from build123d import *

# Parameters (mm, degrees)
BOSS_EXTRUDE1_DEPTH = 7.77


with BuildPart() as part:
    # Sketch1 → Boss-Extrude1 (new body)
    # profile 1 of 5: a face of its own
    with BuildSketch(Plane.XY):
        with BuildLine():
            ThreePointArc((3.404182759, -40.079440399), (3.403839221, -40.127801725), (3.402808675, -40.176153289))
            ThreePointArc((3.402808675, -40.176153289), (5.967670482, -39.875923927), (8.508052822, -39.412122972))
            ThreePointArc((8.508052822, -39.412122972), (35.574552979, -18.977712726), (37.472579791, 14.883150333))
            ThreePointArc((37.472579791, 14.883150333), (36.442962914, 17.251459476), (35.263848757, 19.548999228))
            ThreePointArc((35.263848757, 19.548999228), (30.43912953, 20.428209113), (31.453728524, 25.226283157))
            ThreePointArc((31.453728524, 25.226283157), (29.774333348, 27.188075947), (27.972797119, 29.038337096))
            ThreePointArc((27.972797119, 29.038337096), (18.347193458, 35.903800526), (7.14399719, 39.682057711))
            ThreePointArc((7.14399719, 39.682057711), (4.589484945, 40.057945878), (2.016151733, 40.269560864))
            ThreePointArc((2.016151733, 40.269560864), (2.020874049, 40.165888855), (2.022448638, 40.062121295))
            ThreePointArc((2.022448638, 40.062121295), (-1.382077907, 36.642156299), (-4.817411346, 40.031174701))
            ThreePointArc((-4.817411346, 40.031174701), (-7.369742742, 39.640752918), (-9.891851642, 39.087768817))
            ThreePointArc((-9.891851642, 39.087768817), (-34.597565404, 20.705334291), (-39.122221714, -9.7546998))
            ThreePointArc((-39.122221714, -9.7546998), (-38.417536694, -12.239087971), (-37.555259765, -14.673270392))
            ThreePointArc((-37.555259765, -14.673270392), (-34.193471955, -14.769982316), (-32.539881663, -17.698567233))
            ThreePointArc((-32.539881663, -17.698567233), (-33.081813677, -19.546068243), (-34.535867272, -20.808081887))
            ThreePointArc((-34.535867272, -20.808081887), (-33.133010631, -22.976205225), (-31.594239644, -25.05007827))
            ThreePointArc((-31.594239644, -25.05007827), (-21.298252211, -34.235754012), (-8.508052822, -39.412122972))
            ThreePointArc((-8.508052822, -39.412122972), (-5.967670482, -39.875923927), (-3.402808675, -40.176153289))
            ThreePointArc((-3.402808675, -40.176153289), (-0.048361325, -36.675601178), (3.404182759, -40.079440399))
        make_face()
        with BuildLine():
            ThreePointArc((-22.494419384, -11.066975129), (-5.681299846, 24.417200372), (25.069440399, 0))
            ThreePointArc((25.069440399, 0), (5.681299846, -24.417200372), (-22.494419384, -11.066975129))
        make_face(mode=Mode.SUBTRACT)
    # profile 2 of 5: a face of its own
    with BuildSketch(Plane.XY):
        with BuildLine():
            ThreePointArc((35.263848757, 19.548999228), (36.442962914, 17.251459476), (37.472579791, 14.883150333))
            ThreePointArc((37.472579791, 14.883150333), (40.378310636, 27.098559849), (27.972797119, 29.038337096))
            ThreePointArc((27.972797119, 29.038337096), (29.774333348, 27.188075947), (31.453728524, 25.226283157))
            ThreePointArc((31.453728524, 25.226283157), (34.9303084, 25.328891825), (36.69889556, 22.334023609))
            ThreePointArc((36.69889556, 22.334023609), (36.319038644, 20.767521125), (35.263848757, 19.548999228))
        make_face()
    # profile 3 of 5: a face of its own
    with BuildSketch(Plane.XY):
        with BuildLine():
            ThreePointArc((2.016151733, 40.269560864), (4.589484945, 40.057945878), (7.14399719, 39.682057711))
            ThreePointArc((7.14399719, 39.682057711), (-1.695633435, 48.606923637), (-9.891851642, 39.087768817))
            ThreePointArc((-9.891851642, 39.087768817), (-7.369742742, 39.640752918), (-4.817411346, 40.031174701))
            ThreePointArc((-4.817411346, 40.031174701), (-1.516784191, 43.480042232), (2.016151733, 40.269560864))
        make_face()
    # profile 4 of 5: a face of its own
    with BuildSketch(Plane.XY):
        with BuildLine():
            ThreePointArc((-39.122221714, -9.7546998), (-43.631335255, -21.474193014), (-31.594239644, -25.05007827))
            ThreePointArc((-31.594239644, -25.05007827), (-33.133010631, -22.976205225), (-34.535867272, -20.808081887))
            ThreePointArc((-34.535867272, -20.808081887), (-39.028605211, -19.208850623), (-37.555259765, -14.673270392))
            ThreePointArc((-37.555259765, -14.673270392), (-38.417536694, -12.239087971), (-39.122221714, -9.7546998))
        make_face()
    # profile 5 of 5: a face of its own
    with BuildSketch(Plane.XY):
        with BuildLine():
            ThreePointArc((8.508052822, -39.412122972), (5.967670482, -39.875923927), (3.402808675, -40.176153289))
            ThreePointArc((3.402808675, -40.176153289), (0, -43.483623159), (-3.402808675, -40.176153289))
            ThreePointArc((-3.402808675, -40.176153289), (-5.967670482, -39.875923927), (-8.508052822, -39.412122972))
            ThreePointArc((-8.508052822, -39.412122972), (0, -48.613623159), (8.508052822, -39.412122972))
        make_face()
    extrude(amount=BOSS_EXTRUDE1_DEPTH)

    # Fillet1
    # a fillet whose section is not a circle: 5 mm, written as the material it adds along each edge (its section moved 0.00015 mm through the faces so that the kernel can cut it)
    with BuildSketch(Plane(origin=(27.972797119, 29.038337096, 0), x_dir=(-0.7478052572443031, 0.6639181404644565, 0), z_dir=(0, 0, 1))) as fillet1_piece_1:
        with BuildLine():
            Bezier((3.27455803, 0), (0.443727696, -0.114917188), (-0.912581333, -2.602331942), weights=[1, 0.435020662, 1])
            Line((-0.912581333, -2.602331942), (-1.000377754, -2.554459315))
            ThreePointArc((-1.000377754, -2.554459315), (-0.444974343, -1.30513366), (-0.098468347, 0.017435156))
            Line((-0.098468347, 0.017435156), (0.004065293, 0.099917333))
            ThreePointArc((0.004065293, 0.099917333), (1.637282071, 0.066668632), (3.270501884, 0.099917705))
            Line((3.270501884, 0.099917705), (3.27455803, 0))
        make_face()
    extrude(amount=7.77)
    with BuildSketch(Plane(origin=(37.472579791, 14.883150333, 0), x_dir=(0.7809050051368507, 0.62464980024988, 0), z_dir=(0, 0, 1))) as fillet1_piece_2:
        with BuildLine():
            Bezier((2.757704884, 0), (-0.038396039, -0.456755922), (-1.083618682, -3.090064861), weights=[1, 0.435020662, 1])
            Line((-1.083618682, -3.090064861), (-1.176564622, -3.053172417))
            ThreePointArc((-1.176564622, -3.053172417), (-0.604722781, -1.522973292), (-0.09563314, 0.029228455))
            Line((-0.09563314, 0.029228455), (0.016132368, 0.098690155))
            ThreePointArc((0.016132368, 0.098690155), (1.378851781, -0.011991736), (2.741583111, 0.098691886))
            Line((2.741583111, 0.098691886), (2.757704884, 0))
        make_face()
    extrude(amount=7.77)
    with BuildSketch(Plane(origin=(-9.891851642, 39.087768817, 0), x_dir=(-0.9586545512733944, -0.2845724008452099, 0), z_dir=(0, 0, 1))) as fillet1_piece_3:
        with BuildLine():
            Bezier((3.277172257, 0), (0.444362291, -0.115089718), (-0.911320112, -2.605106418), weights=[1, 0.434946583, 1])
            Line((-0.911320112, -2.605106418), (-0.999146838, -2.557289411))
            ThreePointArc((-0.999146838, -2.557289411), (-0.444170839, -1.306571665), (-0.0984839, 0.017347088))
            Line((-0.0984839, 0.017347088), (0.004068531, 0.099917201))
            ThreePointArc((0.004068531, 0.099917201), (1.63858918, 0.066615488), (3.273112865, 0.099917573))
            Line((3.273112865, 0.099917573), (3.277172257, 0))
        make_face()
    extrude(amount=7.77)
    with BuildSketch(Plane(origin=(7.14399719, 39.682057711, 0), x_dir=(-0.11742410292813261, 0.9930818596931088, 0), z_dir=(0, 0, 1))) as fillet1_piece_4:
        with BuildLine():
            Bezier((2.759906483, 0), (-0.038093802, -0.45744109), (-1.082121081, -3.093359334), weights=[1, 0.434946583, 1])
            Line((-1.082121081, -3.093359334), (-1.175093979, -3.056534883))
            ThreePointArc((-1.175093979, -3.056534883), (-0.603940648, -1.524686137), (-0.095656384, 0.029152292))
            Line((-0.095656384, 0.029152292), (0.016145239, 0.09868805))
            ThreePointArc((0.016145239, 0.09868805), (1.379952571, -0.012171692), (2.743771831, 0.098689782))
            Line((2.743771831, 0.098689782), (2.759906483, 0))
        make_face()
    extrude(amount=7.77)
    with BuildSketch(Plane(origin=(-39.122221714, -9.7546998, 0), x_dir=(-0.8572531161014109, -0.5148952271427859, 0), z_dir=(0, 0, 1))) as fillet1_piece_5:
        with BuildLine():
            Bezier((2.757951127, 0), (-0.038361657, -0.456825585), (-1.083457749, -3.090421787), weights=[1, 0.435012441, 1])
            Line((-1.083457749, -3.090421787), (-1.176406599, -3.053536679))
            ThreePointArc((-1.176406599, -3.053536679), (-0.604638694, -1.523158848), (-0.095635652, 0.029220234))
            Line((-0.095635652, 0.029220234), (0.016133572, 0.098689958))
            ThreePointArc((0.016133572, 0.098689958), (1.378974902, -0.012010201), (2.741828149, 0.09869169))
            Line((2.741828149, 0.09869169), (2.757951127, 0))
        make_face()
    extrude(amount=7.77)
    with BuildSketch(Plane(origin=(-31.594239644, -25.05007827, 0), x_dir=(-0.9309287843318478, -0.36520076465203083, 0), z_dir=(0, 0, 1))) as fillet1_piece_6:
        with BuildLine():
            Bezier((2.757951127, 0), (-0.038361657, 0.456825585), (-1.083457749, 3.090421787), weights=[1, 0.435012441, 1])
            Line((-1.083457749, 3.090421787), (-1.176406599, 3.053536679))
            ThreePointArc((-1.176406599, 3.053536679), (-0.604638694, 1.523158848), (-0.095635652, -0.029220234))
            Line((-0.095635652, -0.029220234), (0.016133572, -0.098689958))
            ThreePointArc((0.016133572, -0.098689958), (1.378974902, 0.012010201), (2.741828149, -0.09869169))
            Line((2.741828149, -0.09869169), (2.757951127, 0))
        make_face()
    extrude(amount=7.77)
    with BuildSketch(Plane(origin=(-8.508052822, -39.412122972, 0), x_dir=(0.08389843348969565, -0.9964743111881886, 0), z_dir=(0, 0, 1))) as fillet1_piece_7:
        with BuildLine():
            Bezier((2.756625198, 0), (-0.038622025, -0.457301683), (-1.083539201, -3.089920144), weights=[1, 0.435048815, 1])
            Line((-1.083539201, -3.089920144), (-1.17648552, -3.053028659))
            ThreePointArc((-1.17648552, -3.053028659), (-0.604686345, -1.522900359), (-0.095633323, 0.029227856))
            Line((-0.095633323, 0.029227856), (0.016155935, 0.0986863))
            ThreePointArc((0.016155935, 0.0986863), (1.378311931, -0.012113558), (2.740479863, 0.098688034))
            Line((2.740479863, 0.098688034), (2.756625198, 0))
        make_face()
    extrude(amount=7.77)
    with BuildSketch(Plane(origin=(8.508052822, -39.412122972, 0), x_dir=(0.968097352048771, 0.25057437410109984, 0), z_dir=(0, 0, 1))) as fillet1_piece_8:
        with BuildLine():
            Bezier((3.274395165, 0), (0.444318442, -0.114880859), (-0.912202503, -2.601320641), weights=[1, 0.435048815, 1])
            Line((-0.912202503, -2.601320641), (-0.999987888, -2.553427781))
            ThreePointArc((-0.999987888, -2.553427781), (-0.444669934, -1.304668221), (-0.098472652, 0.017410827))
            Line((-0.098472652, 0.017410827), (0.004065091, 0.099917341))
            ThreePointArc((0.004065091, 0.099917341), (1.637200639, 0.066671941), (3.270339221, 0.099917713))
            Line((3.270339221, 0.099917713), (3.274395165, 0))
        make_face()
    extrude(amount=7.77)


solid = part.part
Model file for the job. Use its own axes, mm. Coordinates: 2 decimals unless noted, no trailing zeros. Write each loop counter-clockwise with the first axis right and the second up, starting at its lowest first coordinate (ties: lowest second). Pieces come first, ordered by that corner, then holes. Notation, with made-up numbers: (25, 79.25) - (76, 79.25) arc R36 cw to (76, 118.25) - close; hole circle Ø10 at (-37, 86). An arc over 180 degrees is marked (long way). Write each question's results on one line, items separated by ' | '. Start each with the question number.
1) Cut at C-C (x = 0). Write the cut outline in (y, z).
2) Cut at D-D (z = 5.75). Count the separate pieces of the cut face and the enclosed holes in it, then the cut area to 3 significant figures.
3) Cut at A-A (x = 14). Write the cut outline in (y, z), then the cut area to 3 significant figures.
4) Flat gauge pins, fed straight in: P1, Ø1, axis at x = 4.5, y = 22.5, coming from the +Z side; P2, Ø1.5, axis at y = -16.5, z = 4, coming from the +X side; P3, Ø3, axis at x = -14.5, z = 3, coming from the +Y side. Where does each tip first touch, or does it go through?
5) Probe line 1 along Y through (x, z) = (0, 3.75); line 2 along Y through (x, z) = (-4.5, 0.5); line 3 along Y through (x, z) = (-37, 4.75). List the from-to ranges inside material, lowest first. Write a range as from..to.
6) Cut at B-B (y = -5). Write the cut outline in (x, z), then the cut area to 3 significant figures.
Returned:
1) outline: (-48.61, 0) - (-43.48, 0) - (-43.48, 7.77) - (-48.61, 7.77) - close; (-36.68, 0) - (-25.07, 0) - (-25.07, 7.77) - (-36.68, 7.77) - close; (25.07, 0) - (36.94, 0) - (36.94, 7.77) - (25.07, 7.77) - close; (43.18, 0) - (48.5, 0) - (48.5, 7.77) - (43.18, 7.77) - close
2) separate pieces: 1 | enclosed holes: 5 | area: 3,470 mm^2
3) outline: (-37.81, 0) - (-20.8, 0) - (-20.8, 7.77) - (-37.81, 7.77) - close; (20.8, 0) - (37.81, 0) - (37.81, 7.77) - (20.8, 7.77) - close | area: 264 mm^2
4) P1: through | P2: x = 37.12 | P3: y = 38.17
5) line 1: -48.61..-43.48, -36.68..-25.07, 25.07..36.94, 43.18..48.5 | line 2: -47.33..-24.66, 24.66..38.62, 41.5..48.03 | line 3: -26.19..-20.96, -14.44..16.02
6) outline: (-40.01, 0) - (-24.57, 0) - (-24.57, 7.77) - (-40.01, 7.77) - close; (24.57, 0) - (40.01, 0) - (40.01, 7.77) - (24.57, 7.77) - close | area: 240 mm^2
